The drawing under review shows one solid part. Ordinate dimensions are in mm from its lowest x, y, z. Coordinates: 2 decimals unless noted, no trailing zeros. Write each loop counter-clockwise with the first axis right and the second up, starting at its lowest first coordinate (ties: lowest second). Pieces come first, ordered by that corner, then holes. Notation, with made-up numbers: (28.25, -23.5) - (73.25, -23.5) arc R7 ccw to (73.25, -16.5) - close; hole circle Ø8 at (50, -7.5). An arc over 180 degrees is marked (long way). Use a Markdown table: item, result.
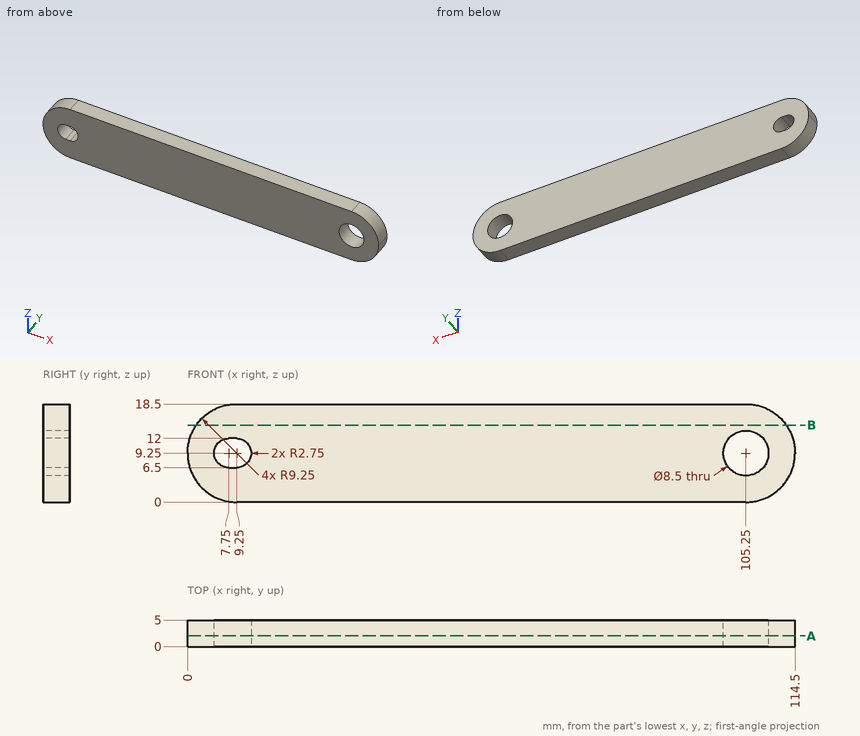
(1) For pin 1 (1.6 mm diameter, centred on x = 8.5, y = 1.5, fed in from -Z); pin 2 (2 mm diameter, centred on y = 3, z = 7, fed in from +X) (3 decimals); pin 3 (1.6 mm diameter, centred on x = 8, y = 3, fed in from +Z), all flat-tipped, find the tip position at first contact; note any pin that passes through.
Determined:
| item | result |
|---|---|
| pin 1 | z = 0 |
| pin 2 | x = 114.415 |
| pin 3 | z = 18.49 |
(2) For L1, parallel to Z at x = 105.25, y = 3.7; L2, parallel to X at y = 3.1, z = 7.75 (1 decimal); L3, parallel to X at y = 3.05, z = 15.75, list the stretches that pass through material, from the lowest coordinate up. Write a range as from..to.
Determined:
| item | result |
|---|---|
| L1 | 0..5, 13.5..18.5 |
| L2 | 0.1..5.4, 11.6..101.3, 109.2..114.4 |
| L3 | 2.67..111.83 |
(3) Take a section at A-A on y = 2.05. State how many separate pieces and enclosed holes the cut face has, and give its area (3 significant figures).
Determined:
| item | result |
|---|---|
| separate pieces | 1 |
| enclosed holes | 2 |
| area | 1,960 mm2 |
(4) Take a section at B-B on z = 14.5. Write out the cut boundary in (x, y), and give its area (3 significant figures).
Determined:
| item | result |
|---|---|
| outline | (1.63, 0) - (112.87, 0) - (112.87, 5) - (1.63, 5) - close |
| area | 556 mm2 |
